from build123d import *

# Parameters (mm, degrees)
BOSS_EXTRUDE1_DEPTH = 20
SKETCH2_W           = 9
SKETCH2_H           = 6
BOSS_EXTRUDE2_DEPTH = 8
CHAMFER1_SIZE       = 3.5
CHAMFER1_SIZE2      = 7.5
SKETCH3_R           = 1.5
CUT_EXTRUDE1_DEPTH  = 44.597859544
SKETCH3_3_R         = 2.6
SKETCH3_3_R_2       = 1.5
CUT_EXTRUDE2_DEPTH  = 1.5
FILLET1_R           = 4


with BuildPart() as part:
    # Sketch1 → Boss-Extrude1 (new body)
    with BuildSketch(Plane(origin=(0, 0, 0), x_dir=(0, 0, -1), z_dir=(1, 0, 0))):
        with BuildLine():
            Line((0, 0), (7.140740034, 5))
            Line((7.140740034, 5), (24.410086433, 5))
            Line((24.410086433, 5), (25.410086433, 5))
            ThreePointArc((25.410086433, 5), (28.945620339, 3.535533906), (30.410086433, 0))
            Line((30.410086433, 0), (30.410086433, -11))
            Line((30.410086433, -11), (24.410086433, -11))
            Line((24.410086433, -11), (24.410086433, 0))
            Line((24.410086433, 0), (0, 0))
        make_face()
    extrude(amount=BOSS_EXTRUDE1_DEPTH)

    # Sketch2 → Boss-Extrude2 (add)
    with BuildSketch(Plane.XZ.offset(11)):
        with Locations((15.5, -27.410086433)):
            Rectangle(SKETCH2_W, SKETCH2_H)
        with Locations((4.5, -27.410086433)):
            Rectangle(SKETCH2_W, SKETCH2_H)
    extrude(amount=BOSS_EXTRUDE2_DEPTH)

    # Chamfer1
    chamfer1_edges = [part.edges().sort_by_distance(p)[0] for p in [
        (10, 0, -24.410086433),
    ]]
    chamfer1_side = [part.faces().sort_by_distance(p)[0] for p in [
        (10, 0, -12.205043216),
    ]]
    chamfer(chamfer1_edges, length=CHAMFER1_SIZE, length2=CHAMFER1_SIZE2, reference=chamfer1_side[0])

    # Sketch3 → Cut-Extrude1 (cut, through all)
    with BuildSketch(Plane(origin=(0, 5, 0), x_dir=(1, 0, 0), z_dir=(0, 1, 0))):
        with Locations(Location((10, 15.150730497, 0), (0, 0, 270))):
            Circle(SKETCH3_R)
    extrude(amount=-CUT_EXTRUDE1_DEPTH, mode=Mode.SUBTRACT)

    # Sketch3_3 → Cut-Extrude2 (cut)
    with BuildSketch(Plane(origin=(0, 5, 0), x_dir=(1, 0, 0), z_dir=(0, 1, 0))):
        with Locations(Location((10, 15.150730497, 0), (0, 0, 270))):
            Circle(SKETCH3_3_R)
        with Locations(Location((10, 15.150730497, 0), (0, 0, 270))):
            Circle(SKETCH3_3_R_2, mode=Mode.SUBTRACT)
    extrude(amount=-CUT_EXTRUDE2_DEPTH, mode=Mode.SUBTRACT)

    # Fillet1
    fillet1_edges = [part.edges().sort_by_distance(p)[0] for p in [
        (0, -9.5, -30.410086433),
        (20, -9.5, -30.410086433),
        (20, 3.535533906, -28.945620339),
        (20, 5, -16.275413233),
        (0, 5, -16.275413233),
        (0, 3.535533906, -28.945620339),
    ]]
    fillet(fillet1_edges, radius=FILLET1_R)


solid = part.part
Source: CAD feature listing. Evaluate the final solid. Frame: model axes, mm. A direction names the side the tool comes from. Give positions to 0.01 mm unless a question says otherwise; leave off trailing zeros. Write each loop counter-clockwise with the first axis right and the second up, starting at its lowest first coordinate (ties: lowest second). Pieces come first, ordered by that corner, then holes. Notation, with made-up numbers: M 66.25,66.25 L 90.25,66.25 A20 ccw 90.25,70.25 Z; hole C 53,-35.75 d8. An arc over 180 degrees is marked long. Answer as a JSON object with one key per item and string values.
Q1. Cut plane B-B, the plane x = 10. Return the cut outline in (y, z), then the cut area to 3 significant figures.
Geometry check:
{"outline": "M -11,-30.41 L 0,-30.41 A5 ccw 5,-25.41 L 5,-17.75 L 3.5,-17.75 L 3.5,-16.65 L 0,-16.65 L 0,-20.91 L -7.5,-24.41 L -11,-24.41 Z; M 0,-13.65 L 3.5,-13.65 L 3.5,-12.55 L 5,-12.55 L 5,-7.14 L 0,0 Z", "area": "190 mm^2"}
Q2. Ray query, line 1 along X through (y, z) = (-17, -25); line 2 along Y through (x, z) = (16, -18); line 3 along Z through (x, y) = (15.75, -10.5). Return the intervals inside material, ascending.
Geometry check:
{"line 1": "x = 0 to 9, 11 to 20", "line 2": "y = 0 to 5", "line 3": "z = -30.41 to -24.41"}
Q3. Cut plane A-A, the plane y = -16.25. Return the cut outline in (x, z), then the cut area to 3 significant figures.
Geometry check:
{"outline": "M 0,-26.41 A4 ccw 4,-30.41 L 9,-30.41 L 9,-24.41 L 0,-24.41 Z; M 11,-30.41 L 16,-30.41 A4 ccw 20,-26.41 L 20,-24.41 L 11,-24.41 Z", "area": "101 mm^2"}
Q4. Contact query for flat-ended pins moving along their axis: P1, Ø1.6, axis at x = 11, z = -16.5, coming from the +Y side; P2, Ø10, axis at x = 2.5, y = 1, coming from the -Z side; P3, Ø0.6, axis at x = 9.5, z = -27, coming from the -Y side; P4, Ø2, axis at x = 7.5, y = -9.5, coming from the +Z side. Output: stop coordinate, or through.
Geometry check:
{"P1": "stops at y = 3.5", "P2": "stops at z = -30.41", "P3": "stops at y = -11", "P4": "stops at z = -24.41"}
Q5. Cut plane D-D, the plane z = -7.5. Return the cut outline in (x, y), then the cut area to 3 significant figures.
Geometry check:
{"outline": "M 0,0 L 20,0 L 20,1 A4 ccw 16,5 L 4,5 A4 ccw 0,1 Z", "area": "93.1 mm^2"}
Q6. Access query for faces 1 (the face through (12, -13, -24.41)), 2 (the face through (7.46, 4.26, -15.71)), 3 (the face through (9, -15, -27)). Directions: +Z, -Z, +X, -X, +Y, -Y. A direction counts if a zero-diameter tool reaches every point of the face in a straight line with its end or side. Return the directions, or none.
Geometry check:
{"face 1": "+Z, +X, -X, -Y", "face 2": "+Y", "face 3": "+Z, -Z, -Y"}
Q7. Cut plane C-C, the plane x = 14.5. Return the cut outline in (y, z), then the cut area to 3 significant figures.
Geometry check:
{"outline": "M -19,-30.41 L 0,-30.41 A5 ccw 5,-25.41 L 5,-7.14 L 0,0 L 0,-20.91 L -7.5,-24.41 L -19,-24.41 Z", "area": "256 mm^2"}
